```python
from build123d import *

# Parameters (mm, degrees)
F0_W     = 120
F0_H     = 80
F0_W_2   = 100
F0_H_2   = 60
F1_DEPTH = 15
F2_R     = 3.2
F3_DEPTH = 10.001
F4_SIZE  = 3


with BuildPart() as f1:
    # F0 (on Top) → F1 (new body)
    with BuildSketch(Plane.XY):
        with Locations((-60, 40)):
            Rectangle(F0_W, F0_H)
        with Locations((-60, 40)):
            Rectangle(F0_W_2, F0_H_2, mode=Mode.SUBTRACT)
    extrude(amount=F1_DEPTH)

    # F2 (on face) → F3 (cut, through all)
    with BuildSketch(Plane(origin=(0, 10, 0), x_dir=(-1, 0, 0), z_dir=(0, 1, 0))):
        with Locations((72.5, 7.5)):
            Circle(F2_R)
        with Locations((47.5, 7.5)):
            Circle(F2_R)
        with Locations((97.5, 7.5)):
            Circle(F2_R)
        with Locations((22.5, 7.5)):
            Circle(F2_R)
    extrude(amount=-F3_DEPTH, mode=Mode.SUBTRACT)

    # F4
    f4_edges = [f1.edges().sort_by_distance(p)[0] for p in [
        (-60, 0, 15),
        (0, 40, 15),
        (-60, 80, 15),
        (-120, 40, 15),
        (-10, 40, 15),
        (-60, 10, 15),
        (-110, 40, 15),
        (-60, 70, 15),
        (-60, 0, 0),
        (0, 40, 0),
        (-60, 80, 0),
        (-120, 40, 0),
        (-10, 40, 0),
        (-60, 10, 0),
        (-110, 40, 0),
        (-60, 70, 0),
    ]]
    chamfer(f4_edges, length=F4_SIZE)


solid = f1.part
```
CAD build for the part. Positions are in the model's coordinates, mm. A direction names the side the tool comes from. Round coordinates to 2 decimals unless told otherwise and drop trailing zeros. Order: outer loops, then holes, each group sorted by start corner. A loop starts at its lowest first (then second) coordinate and runs counter-clockwise, first axis right, second up. Notation, with made-up numbers: (70.25, -32.75) - (99.25, -32.75) arc R17 ccw to (99.25, -0.75) - close; hole circle Ø11 at (81, 15). An arc over 180 degrees is marked (long way). Answer in a Markdown table with one row per item. Add a question column.
(1) Drop flat-ended pins along their axis: pin 1 Ø7 at (x, z) = (-51.5, 8.5) entering from -Y; pin 2 Ø4 at (x, z) = (-47.5, 7.5) entering from -Y. Give the stop position or say it passes through.
(2) Band-saw the part on C-C on z = 13.25. List the corners of the cut face in (x, y), and give its area (3 significant figures).
(3) Band-saw the part on D-D on z = 7.5. List the corners of the cut face in (x, y).
(4) Band-saw the part on B-B on x = -61. List the corners of the cut face in (y, z), and give its area (3 significant figures).
(5) Band-saw the part on A-A on y = 47. List the corners of the cut face in (x, z), and give its area (3 significant figures).
(6) Mould opens along Z. For faces 4 (the face through (-61, 9, 2)), 5 (the face through (-73.977, 5.07, 4.661)), 6 (the face through (-61, 2, 14)) say: +Z half, -Z half, draft (parallel to the pull), parting line (faces both ways), or undercut.
(7) Probe L1, parallel to X at y = 59.5, z = 10; L2, parallel to Y at x = -37, z = 8.5; L3, parallel to Z at x = -72.5, y = 4. List the from-to ranges inside material, lowest first. Write a range as [from, to].
(8) 3-axis set-ups, long thin cutter, end or side, ignore diameter. For faces 1 (the face through (-48.977, 5.07, 4.661)), 2 (the face through (-61, 70, 7)), 3 (the face through (-111, 40, 2)): which of +Z, -Z, +X, -X, +Y, -Y reach the whole face in a straight line?
Data:
| question | item | result |
|---|---|---|
| 1 | pin 1 | stops at y = 0 |
| 1 | pin 2 | stops at y = 70 |
| 2 | outline | (-118.75, 1.25) - (-1.25, 1.25) - (-1.25, 78.75) - (-118.75, 78.75) - close; hole (-111.25, 8.75) - (-8.75, 8.75) - (-8.75, 71.25) - (-111.25, 71.25) - close |
| 2 | area | 2,700 mm^2 |
| 3 | outline | (-120, 0) - (-100.7, 0) - (-100.7, 10) - (-110, 10) - (-110, 70) - (-10, 70) - (-10, 10) - (-19.3, 10) - (-19.3, 0) - (0, 0) - (0, 80) - (-120, 80) - close; (-94.3, 0) - (-75.7, 0) - (-75.7, 10) - (-94.3, 10) - close; (-69.3, 0) - (-50.7, 0) - (-50.7, 10) - (-69.3, 10) - close; (-44.3, 0) - (-25.7, 0) - (-25.7, 10) - (-44.3, 10) - close |
| 4 | outline | (0, 3) - (3, 0) - (7, 0) - (10, 3) - (10, 12) - (7, 15) - (3, 15) - (0, 12) - close; (70, 3) - (73, 0) - (77, 0) - (80, 3) - (80, 12) - (77, 15) - (73, 15) - (70, 12) - close |
| 4 | area | 264 mm^2 |
| 5 | outline | (-120, 3) - (-117, 0) - (-113, 0) - (-110, 3) - (-110, 12) - (-113, 15) - (-117, 15) - (-120, 12) - close; (-10, 3) - (-7, 0) - (-3, 0) - (0, 3) - (0, 12) - (-3, 15) - (-7, 15) - (-10, 12) - close |
| 5 | area | 264 mm^2 |
| 6 | face 4 | -Z half |
| 6 | face 5 | undercut |
| 6 | face 6 | +Z half |
| 7 | L1 | x = [-120, -110], [-10, 0] |
| 7 | L2 | y = [0, 10], [70, 80] |
| 7 | L3 | z = [0, 4.3], [10.7, 15] |
| 8 | face 1 | -Y |
| 8 | face 2 | +Z, -Z |
| 8 | face 3 | -Z |
